Model file for the job. Use its own axes, mm. Coordinates: 2 decimals unless noted, no trailing zeros. Write each loop counter-clockwise with the first axis right and the second up, starting at its lowest first coordinate (ties: lowest second). Pieces come first, ordered by that corner, then holes. Notation, with made-up numbers: M -19,-11 L 2,-11 A33 cw 2,27 Z; hole C 55.5,-36.5 d9. An arc over 180 degrees is marked long. One line per question, with ' | ' between items. Start each with the question number.
(1) Flat gauge pins, fed straight in: pin 1 Ø4 at (x, y) = (127, 363.5) entering from -Z; pin 2 Ø4 at (x, z) = (40, 10) entering from -Y; pin 3 Ø2 at (x, y) = (71.5, 259.5) entering from -Z; pin 4 Ø5 at (x, y) = (160, 261) entering from -Z. Where does each tip first touch, or does it go through?
(2) Cut at A-A (y = 356.5). Write the cut outline in (x, z).
(3) Wall check: probe 1 along Z at (x, y) = (120, 32); probe 2 along Y at (x, z) = (163.5, 7); probe 3 along X at (y, z) = (341.5, 17.25). Give the ranges that are in metal, low to high.
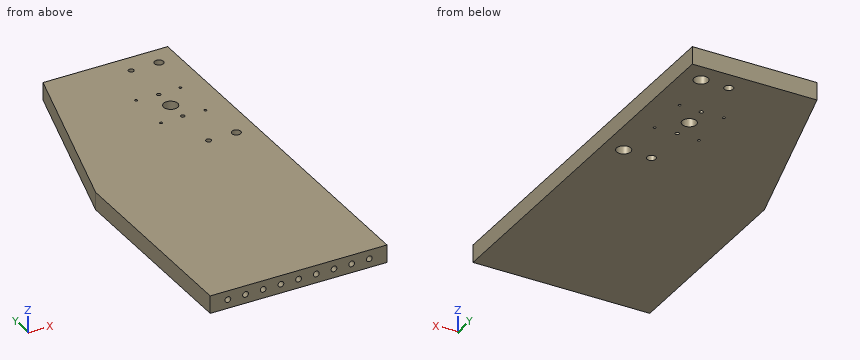
from build123d import *

# Parameters (mm, degrees)
SKETCH1_R                  = 8
SKETCH1_R_2                = 5
SKETCH1_R_3                = 2.25
SKETCH1_R_4                = 1.5
SKETCH1_R_5                = 3
EXTRUDE1_DEPTH             = 20
CUT_EXTRUDE1_START         = -10
CUT_EXTRUDE1_OUTLINE_R     = 8
CUT_EXTRUDE1_OUTLINE_R_2   = 5
CUT_EXTRUDE1_DEPTH         = 10
CUT_EXTRUDE1_START_2       = -6
CUT_EXTRUDE1_2_OUTLINE_R   = 5
CUT_EXTRUDE1_2_OUTLINE_R_2 = 3
CUT_EXTRUDE1_2_DEPTH       = 6
CUT_EXTRUDE1_3_OUTLINE_R   = 3.25
CUT_EXTRUDE1_3_DEPTH       = 60


# Read off the part's stored shape, not the designer's step: Cut-Extrude1
with BuildPart() as part:
    # Sketch1 → Extrude1 (new body)
    with BuildSketch(Plane.XY):
        Polygon((38.999908, 439.49994136), (-20, 229.49994136), (-20, 0), (180, 0), (180, 20), (180, 439.50001453), align=None)
        with Locations((126.999908, 339.49994136)):
            Circle(SKETCH1_R, mode=Mode.SUBTRACT)
        with Locations((157.49992067, 416.99997068)):
            Circle(SKETCH1_R_2, mode=Mode.SUBTRACT)
        with Locations((126.999908, 363.49994136)):
            Circle(SKETCH1_R_3, mode=Mode.SUBTRACT)
        with Locations((126.999908, 315.49994136)):
            Circle(SKETCH1_R_3, mode=Mode.SUBTRACT)
        with Locations((157.49992067, 261.99991204)):
            Circle(SKETCH1_R_2, mode=Mode.SUBTRACT)
        with Locations((151.999908, 364.49994136)):
            Circle(SKETCH1_R_4, mode=Mode.SUBTRACT)
        with Locations((151.999908, 314.49994136)):
            Circle(SKETCH1_R_4, mode=Mode.SUBTRACT)
        with Locations((101.999908, 364.49994136)):
            Circle(SKETCH1_R_4, mode=Mode.SUBTRACT)
        with Locations((101.999908, 314.49994136)):
            Circle(SKETCH1_R_4, mode=Mode.SUBTRACT)
        with Locations((126.12492067, 416.99997068)):
            Circle(SKETCH1_R_5, mode=Mode.SUBTRACT)
        with Locations((126.12492067, 261.99991204)):
            Circle(SKETCH1_R_5, mode=Mode.SUBTRACT)
    extrude(amount=EXTRUDE1_DEPTH)

    # Cut-Extrude1 outline → Cut-Extrude1 (cut)
    # profile 1 of 2: a face of its own
    with BuildSketch(Plane(origin=(0, 0, 0), x_dir=(-1, 0, 0), z_dir=(0, 0, -1)).offset(CUT_EXTRUDE1_START)):
        with Locations((-157.49992067, 416.99997068)):
            Circle(CUT_EXTRUDE1_OUTLINE_R)
        with Locations((-157.49992067, 416.99997068)):
            Circle(CUT_EXTRUDE1_OUTLINE_R_2, mode=Mode.SUBTRACT)
    # profile 2 of 2: a face of its own
    with BuildSketch(Plane(origin=(0, 0, 0), x_dir=(-1, 0, 0), z_dir=(0, 0, -1)).offset(CUT_EXTRUDE1_START)):
        with Locations((-157.49992067, 261.99991204)):
            Circle(CUT_EXTRUDE1_OUTLINE_R)
        with Locations((-157.49992067, 261.99991204)):
            Circle(CUT_EXTRUDE1_OUTLINE_R_2, mode=Mode.SUBTRACT)
    extrude(amount=CUT_EXTRUDE1_DEPTH, mode=Mode.SUBTRACT)

    # Cut-Extrude1 2 outline → Cut-Extrude1 2 (cut)
    # profile 1 of 2: a face of its own
    with BuildSketch(Plane(origin=(0, 0, 0), x_dir=(-1, 0, 0), z_dir=(0, 0, -1)).offset(CUT_EXTRUDE1_START_2)):
        with Locations((-126.12492067, 416.99997068)):
            Circle(CUT_EXTRUDE1_2_OUTLINE_R)
        with Locations((-126.12492067, 416.99997068)):
            Circle(CUT_EXTRUDE1_2_OUTLINE_R_2, mode=Mode.SUBTRACT)
    # profile 2 of 2: a face of its own
    with BuildSketch(Plane(origin=(0, 0, 0), x_dir=(-1, 0, 0), z_dir=(0, 0, -1)).offset(CUT_EXTRUDE1_START_2)):
        with Locations((-126.12492067, 261.99991204)):
            Circle(CUT_EXTRUDE1_2_OUTLINE_R)
        with Locations((-126.12492067, 261.99991204)):
            Circle(CUT_EXTRUDE1_2_OUTLINE_R_2, mode=Mode.SUBTRACT)
    extrude(amount=CUT_EXTRUDE1_2_DEPTH, mode=Mode.SUBTRACT)

    # Cut-Extrude1 3 outline → Cut-Extrude1 3 (cut)
    with BuildSketch(Plane(origin=(0, 0, 0), x_dir=(1, 0, 0), z_dir=(0, 1, 0))):
        with Locations((20, -10)):
            Circle(CUT_EXTRUDE1_3_OUTLINE_R)
        with Locations((40, -10)):
            Circle(CUT_EXTRUDE1_3_OUTLINE_R)
        with Locations((60, -10)):
            Circle(CUT_EXTRUDE1_3_OUTLINE_R)
        with Locations((80, -10)):
            Circle(CUT_EXTRUDE1_3_OUTLINE_R)
        with Locations((100, -10)):
            Circle(CUT_EXTRUDE1_3_OUTLINE_R)
        with Locations((120, -10)):
            Circle(CUT_EXTRUDE1_3_OUTLINE_R)
        with Locations((140, -10)):
            Circle(CUT_EXTRUDE1_3_OUTLINE_R)
        with Locations((160, -10)):
            Circle(CUT_EXTRUDE1_3_OUTLINE_R)
        with Locations((0, -10)):
            Circle(CUT_EXTRUDE1_3_OUTLINE_R)
    extrude(amount=CUT_EXTRUDE1_3_DEPTH, mode=Mode.SUBTRACT)


solid = part.part
Filled in:
1) pin 1: through | pin 2: y = 60 | pin 3: z = 0 | pin 4: z = 10
2) outline: M 15.68,0 L 180,0 L 180,20 L 15.68,20 Z
3) probe 1: 0 to 6.75, 13.25 to 20 | probe 2: 0 to 256.71, 267.29 to 411.71, 422.29 to 439.5 | probe 3: 11.47 to 119.25, 134.75 to 180
